Here's how the part is built. I have some questions about the finished solid (model axes, mm). A direction names the side the tool comes from. Coordinates: 2 decimals unless noted, no trailing zeros. Loops run counter-clockwise (first coordinate to the right, second up) from the corner with the lowest first, then second, coordinate; pieces in that order, holes last. Notation, with made-up numbers: (60, -13.5) - (64, -13.5) arc R12 cw to (64, 9.5) - close; hole circle Ø2 at (-4, -31.5). An arc over 180 degrees is marked (long way). Use a Markdown table: item, result.
```python
from build123d import *

# Parameters (mm, degrees)
SKETCH2_R           = 1.5
SKETCH2_W           = 8.757359312
SKETCH2_H           = 35.757359312
SKETCH2_W_2         = 40
SKETCH2_H_2         = 35.27269061
BOSS_EXTRUDE1_DEPTH = 3
SKETCH2_4_R         = 4.77269061
BOSS_EXTRUDE2_DEPTH = 6
SKETCH2_5_R         = 2.475
SKETCH2_5_R_2       = 4.77269061
BOSS_EXTRUDE3_DEPTH = 10


with BuildPart() as part:
    # Sketch2 → Boss-Extrude1 (new body)
    with BuildSketch(Plane(origin=(0, 0, 0), x_dir=(1, 0, 0), z_dir=(0, 1, 0))):
        Polygon((0, 0), (0, -50), (25, -50), (25, 0), (41.5, 67.785623806), (41.5, 114.52269061), (-16.5, 114.52269061), (-16.5, 67.785623806), align=None)
        with Locations(Location((4.5, -45, 0), (0, 0, 270))):
            Circle(SKETCH2_R, mode=Mode.SUBTRACT)
        with Locations(Location((20.5, -45, 0), (0, 0, 270))):
            Circle(SKETCH2_R, mode=Mode.SUBTRACT)
        with Locations(Location((20.5, -5, 0), (0, 0, 270))):
            Circle(SKETCH2_R, mode=Mode.SUBTRACT)
        with Locations(Location((4.5, -5, 0), (0, 0, 270))):
            Circle(SKETCH2_R, mode=Mode.SUBTRACT)
        Polygon((16.5, 57.25), (28.028914458, 57.25), (16.5, 5.628094968), align=None, mode=Mode.SUBTRACT)
        Polygon((-3.028914458, 57.25), (8.5, 5.628094968), (8.5, 57.25), align=None, mode=Mode.SUBTRACT)
        with Locations((12.5, -25)):
            Rectangle(SKETCH2_W, SKETCH2_H, mode=Mode.SUBTRACT)
        with Locations((12.5, 87.886345305)):
            Rectangle(SKETCH2_W_2, SKETCH2_H_2, mode=Mode.SUBTRACT)
    extrude(amount=BOSS_EXTRUDE1_DEPTH)

    # Sketch2_4 → Boss-Extrude2 (add)
    with BuildSketch(Plane(origin=(0, 0, 0), x_dir=(1, 0, 0), z_dir=(0, 1, 0))):
        with BuildLine():
            Line((-16.385347151, 67.314604722), (-15.349520723, 63.059202262))
            ThreePointArc((-15.349520723, 63.059202262), (-6.641853057, 67.432543142), (-16.385347151, 67.314604722))
        make_face()
        with BuildLine():
            ThreePointArc((41.385347151, 67.314604722), (31.641853057, 67.432543142), (40.349520723, 63.059202262))
            Line((40.349520723, 63.059202262), (41.385347151, 67.314604722))
        make_face()
        with Locations(Location((-11.5, 109.75, 0), (0, 0, 90))):
            Circle(SKETCH2_4_R)
        with Locations(Location((36.5, 109.75, 0), (0, 0, 90))):
            Circle(SKETCH2_4_R)
    extrude(amount=BOSS_EXTRUDE2_DEPTH)

    # Sketch2_5 → Boss-Extrude3 (add)
    # profile 1 of 4: a face of its own
    with BuildSketch(Plane(origin=(0, 0, 0), x_dir=(1, 0, 0), z_dir=(0, 1, 0))):
        with BuildLine():
            Line((-16.385347151, 67.314604722), (-15.349520723, 63.059202262))
            ThreePointArc((-15.349520723, 63.059202262), (-6.641853057, 67.432543142), (-16.385347151, 67.314604722))
        make_face()
        with Locations(Location((-11.5, 66.25, 0), (0, 0, 270))):
            Circle(SKETCH2_5_R, mode=Mode.SUBTRACT)
    # profile 2 of 4: a face of its own
    with BuildSketch(Plane(origin=(0, 0, 0), x_dir=(1, 0, 0), z_dir=(0, 1, 0))):
        with BuildLine():
            ThreePointArc((41.385347151, 67.314604722), (31.641853057, 67.432543142), (40.349520723, 63.059202262))
            Line((40.349520723, 63.059202262), (41.385347151, 67.314604722))
        make_face()
        with Locations(Location((36.5, 66.25, 0), (0, 0, 270))):
            Circle(SKETCH2_5_R, mode=Mode.SUBTRACT)
    # profile 3 of 4: a face of its own
    with BuildSketch(Plane(origin=(0, 0, 0), x_dir=(1, 0, 0), z_dir=(0, 1, 0))):
        with Locations(Location((-11.5, 109.75, 0), (0, 0, 90))):
            Circle(SKETCH2_5_R_2)
        with Locations(Location((-11.5, 109.75, 0), (0, 0, 270))):
            Circle(SKETCH2_5_R, mode=Mode.SUBTRACT)
    # profile 4 of 4: a face of its own
    with BuildSketch(Plane(origin=(0, 0, 0), x_dir=(1, 0, 0), z_dir=(0, 1, 0))):
        with Locations(Location((36.5, 109.75, 0), (0, 0, 90))):
            Circle(SKETCH2_5_R_2)
        with Locations(Location((36.5, 109.75, 0), (0, 0, 270))):
            Circle(SKETCH2_5_R, mode=Mode.SUBTRACT)
    extrude(amount=BOSS_EXTRUDE3_DEPTH)


solid = part.part
```
Q1. I want a section at D-D, the plane z = -75. Write out the boundary of the cut face in (x, y), then the cut area to 3 significant figures.
Check values:
| item | result |
|---|---|
| outline | (-16.5, 0) - (-7.5, 0) - (-7.5, 3) - (-16.5, 3) - close; (32.5, 0) - (41.5, 0) - (41.5, 3) - (32.5, 3) - close |
| area | 54.0 mm^2 |
Q2. I want a section at B-B, the plane x = 1.5. Write out the boundary of the cut face in (y, z).
Check values:
| item | result |
|---|---|
| outline | (0, -114.52) - (3, -114.52) - (3, -105.52) - (0, -105.52) - close; (0, -70.25) - (3, -70.25) - (3, -57.25) - (0, -57.25) - close; (0, -36.97) - (3, -36.97) - (3, 50) - (0, 50) - close |
Q3. Which directions (+Z, -Z, +X, -X, +Y, -Y) give clear straight access to the entire face, cutting with the end or side of a thin tool? Please do faces 4 (the face through (39, 10, -112)), 5 (the face through (31.69, 6.45, -67.61)), 6 (the face through (12, 1, -105.523)).
Check values:
| item | result |
|---|---|
| face 4 | +Z, -Z, +X, -X, +Y |
| face 5 | +Y |
| face 6 | +Y, -Y |
Q4. I want a section at C-C, the plane y = 4.5. Write out the boundary of the cut face in (x, z).
Check values:
| item | result |
|---|---|
| outline | (-16.39, -67.31) arc R5 ccw (long way) to (-15.35, -63.06) - close; circle Ø9.55 at (-11.5, -109.75); circle Ø9.55 at (36.5, -109.75); (40.35, -63.06) arc R5 ccw (long way) to (41.39, -67.31) - close |
Q5. Will these pins go through, and if not, where does the flat tip stop? P1, Ø3.5, axis at y = 2, z = 23.5, coming from the -X side; P2, Ø4, axis at x = 36.5, z = -66.25, coming from the +Y side; P3, Ø2, axis at x = 16, z = -17, coming from the +Y side.
Check values:
| item | result |
|---|---|
| P1 | x = 0 |
| P2 | y = 6 |
| P3 | y = 3 |
Q6. If we mould it in two halves opening along X, with no side actions, what happens to faces 1 (the face through (13, 1, -114.523)), 2 (the face through (16.879, 1, 25)), 3 (the face through (-16.5, 1, -91))? For each: pulls with the +X half, pulls with the -X half, needs draft (parallel to the pull), parting line crosses it, or undercut.
Check values:
| item | result |
|---|---|
| face 1 | needs draft |
| face 2 | undercut |
| face 3 | pulls with the -X half |
Q7. Please list where these lines run through material, in increasing order: L1, parallel to X at y = 0.8, z = 45; L2, parallel to Z at x = 36.5, y = 7.8 (3 decimals); L3, parallel to X at y = 8.7, z = -109.75 (3 decimals). Write a range as from..to.
Check values:
| item | result |
|---|---|
| L1 | 0..3, 6..19, 22..25 |
| L2 | -114.523..-112.225, -107.275..-104.977, -71.25..-68.725, -63.775..-61.25 |
| L3 | -16.273..-13.975, -9.025..-6.727, 31.727..34.025, 38.975..41.273 |
Q8. I want a section at A-A, the plane z = 5. Write out the boundary of the cut face in (x, y).
Check values:
| item | result |
|---|---|
| outline | (0, 0) - (3, 0) - (3, 3) - (0, 3) - close; (6, 0) - (19, 0) - (19, 3) - (6, 3) - close; (22, 0) - (25, 0) - (25, 3) - (22, 3) - close |
